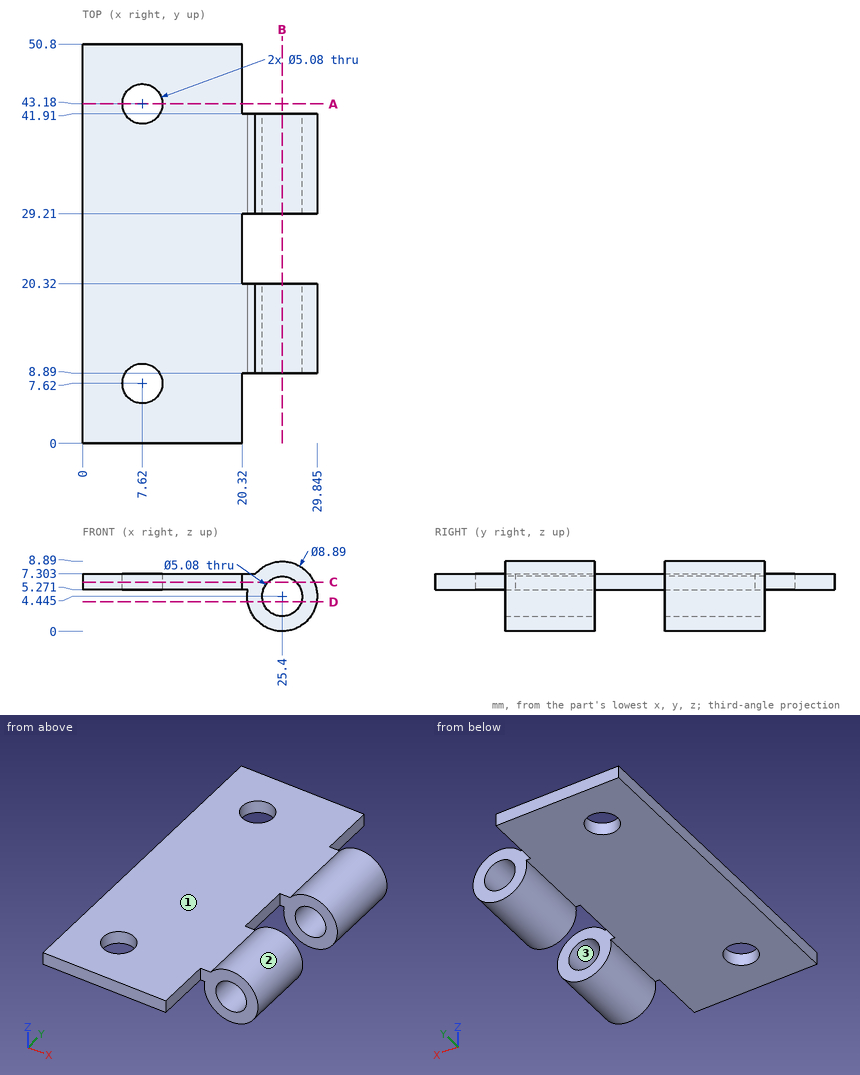
Job drawing, mm, ordinate dimensions from the low corner. One solid piece. Give positions to 0.01 mm unless a question says otherwise; leave off trailing zeros. Order: outer loops, then holes, each group sorted by start corner. A loop starts at its lowest first (then second) coordinate and runs counter-clockwise, first axis right, second up. Notation, with made-up numbers: (31, 6.25) -> (68, 6.25) arc R15 cw to (68, 32.25) -> close; hole circle Ø8 at (77, -8). An arc over 180 degrees is marked (long way). Return JSON: item names as keys, results as strings.
Q1. Flat gauge pins, fed straight in: pin 1 (8 mm diameter, centred on x = 7.62, y = 7.62, fed in from +Z); pin 2 (5 mm diameter, centred on x = 22, z = 2, fed in from -Y); pin 3 (5 mm diameter, centred on y = 43.5, z = 1, fed in from -X); pin 4 (4 mm diameter, centred on x = 8.5, z = 5.5, fed in from -Y). Where does each tip first touch, or does it go through?
Working result:
{"pin 1": "z = 7.3", "pin 2": "y = 8.89", "pin 3": "x = 21.22", "pin 4": "y = 0"}
Q2. Saw through at A-A (y = 43.18). Write the cut outline in (x, z).
Working result:
{"outline": "(0, 5.27) -> (5.08, 5.27) -> (5.08, 7.3) -> (0, 7.3) -> close; (10.16, 5.27) -> (20.32, 5.27) -> (20.32, 7.3) -> (10.16, 7.3) -> close"}
Q3. Mould opens along X. For the marked faces 1, 2 and 3 say: pulls with the +X half, pulls with the -X half, needs draft (parallel to the pull), parting line crosses it, or undercut.
Working result:
{"face 1": "needs draft", "face 2": "parting line crosses it", "face 3": "undercut"}
Q4. Saw through at B-B (x = 25.4). Write the cut outline in (y, z) (1 decimal).
Working result:
{"outline": "(8.9, 0) -> (20.3, 0) -> (20.3, 1.9) -> (8.9, 1.9) -> close; (8.9, 7) -> (20.3, 7) -> (20.3, 8.9) -> (8.9, 8.9) -> close; (29.2, 0) -> (41.9, 0) -> (41.9, 1.9) -> (29.2, 1.9) -> close; (29.2, 7) -> (41.9, 7) -> (41.9, 8.9) -> (29.2, 8.9) -> close"}
Q5. Drill centre lines: line 1 (Y direction, x = 7.62, z = 6.3); line 2 (Y direction, x = 27.75, z = 1); line 3 (Z direction, x = 20.25, y = 3). Where is each one in solid material? Low to high.
Working result:
{"line 1": "0 to 5.08, 10.16 to 40.64, 45.72 to 50.8", "line 2": "8.89 to 20.32, 29.21 to 41.91", "line 3": "5.27 to 7.3"}
Q6. Saw through at D-D (z = 3.75). Write the cut outline in (x, y).
Working result:
{"outline": "(21.01, 8.89) -> (22.96, 8.89) -> (22.96, 20.32) -> (21.01, 20.32) -> close; (21.01, 29.21) -> (22.96, 29.21) -> (22.96, 41.91) -> (21.01, 41.91) -> close; (27.84, 8.89) -> (29.79, 8.89) -> (29.79, 20.32) -> (27.84, 20.32) -> close; (27.84, 29.21) -> (29.79, 29.21) -> (29.79, 41.91) -> (27.84, 41.91) -> close"}
Q7. Saw through at C-C (z = 6.25). Write the cut outline in (x, y), then the cut area to 3 significant figures.
Working result:
{"outline": "(0, 0) -> (20.32, 0) -> (20.32, 8.89) -> (23.61, 8.89) -> (23.61, 20.32) -> (20.32, 20.32) -> (20.32, 29.21) -> (23.61, 29.21) -> (23.61, 41.91) -> (20.32, 41.91) -> (20.32, 50.8) -> (0, 50.8) -> close; (27.19, 8.89) -> (29.46, 8.89) -> (29.46, 20.32) -> (27.19, 20.32) -> close; (27.19, 29.21) -> (29.46, 29.21) -> (29.46, 41.91) -> (27.19, 41.91) -> close; hole circle Ø5.08 at (7.62, 7.62); hole circle Ø5.08 at (7.62, 43.18)", "area": "1,130 mm²"}
